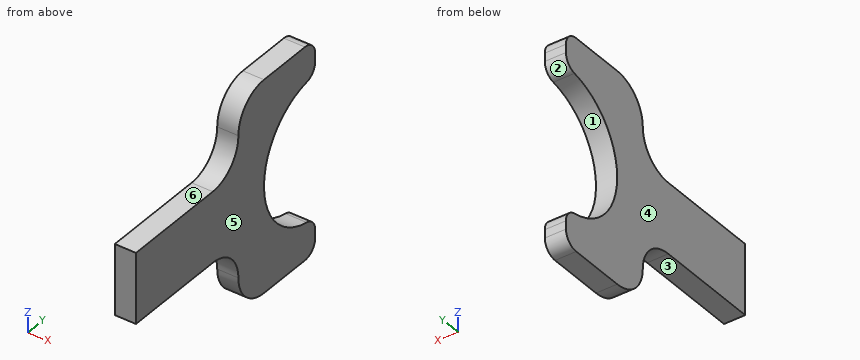
```python
from build123d import *

# Parameters (mm, degrees)
SKETCH1_W           = 30
SKETCH1_H           = 35
BOSS_EXTRUDE1_DEPTH = 3
SKETCH2_W           = 10
SKETCH2_H           = 20
CUT_EXTRUDE1_DEPTH  = 3
SKETCH5_R           = 10
CUT_EXTRUDE2_DEPTH  = 3
FILLET1_DEPTH       = 3
FILLET1_2_DEPTH     = 3
FILLET2_R           = 2


with BuildPart() as part:
    # Sketch1 → Boss-Extrude1 (new body)
    with BuildSketch(Plane(origin=(0, 0, 0), x_dir=(0, 0, -1), z_dir=(1, 0, 0))):
        with Locations((15, 17.5)):
            Rectangle(SKETCH1_W, SKETCH1_H)
    extrude(amount=BOSS_EXTRUDE1_DEPTH)

    # Sketch2 → Cut-Extrude1 (cut)
    with BuildSketch(Plane(origin=(3, 0, 0), x_dir=(0, 0, -1), z_dir=(1, 0, 0))):
        with Locations((5, 10)):
            Rectangle(SKETCH2_W, SKETCH2_H)
        with Locations((25, 10)):
            Rectangle(SKETCH2_W, SKETCH2_H)
    extrude(amount=-CUT_EXTRUDE1_DEPTH, mode=Mode.SUBTRACT)

    # Sketch5 → Cut-Extrude2 (cut)
    with BuildSketch(Plane(origin=(3, 0, 0), x_dir=(0, 0, -1), z_dir=(1, 0, 0))):
        with Locations((15, 35)):
            Circle(SKETCH5_R)
    extrude(amount=-CUT_EXTRUDE2_DEPTH, mode=Mode.SUBTRACT)

    # Fillet1: read off the stored shape, not the designer's step
    # Fillet1 outline → Fillet1 (cut)
    with BuildSketch(Plane.YZ):
        with BuildLine():
            ThreePointArc((25, -30), (21.464466094, -28.535533906), (20, -25))
            Line((20, -25), (20, -30))
            Line((20, -30), (25, -30))
        make_face()
        with BuildLine():
            Line((20, 0), (20, -5))
            ThreePointArc((20, -5), (21.464466094, -1.464466094), (25, 0))
            Line((25, 0), (20, 0))
        make_face()
    extrude(amount=FILLET1_DEPTH, mode=Mode.SUBTRACT)

    # Fillet1 2 outline → Fillet1 2 (add)
    with BuildSketch(Plane.YZ):
        with BuildLine():
            Line((20, -20), (15, -20))
            ThreePointArc((15, -20), (18.535533906, -21.464466094), (20, -25))
            Line((20, -25), (20, -20))
        make_face()
        with BuildLine():
            Line((20, -10), (20, -5))
            ThreePointArc((20, -5), (18.535533906, -8.535533906), (15, -10))
            Line((15, -10), (20, -10))
        make_face()
    extrude(amount=FILLET1_2_DEPTH)

    # Fillet2
    fillet2_edges = [part.edges().sort_by_distance(p)[0] for p in [
        (1.5, 35, -25),
        (1.5, 35, -5),
        (1.5, 35, 0),
        (1.5, 35, -30),
    ]]
    fillet(fillet2_edges, radius=FILLET2_R)


solid = part.part
```
Geometry check sheet. Reference: the model listing, model coordinates, mm. Face numbers are marked on the shaded views. A direction names the side the tool comes from. Round coordinates to 2 decimals unless told otherwise and drop trailing zeros. Loops run counter-clockwise (first coordinate to the right, second up) from the corner with the lowest first, then second, coordinate; pieces in that order, holes last. Notation, with made-up numbers: (37, 19) - (72, 19) arc R32 cw to (72, 57) - close; hole circle Ø4 at (32.25, 45). An arc over 180 degrees is marked (long way). Write each question's results on one line, items separated by ' | '. Start each with the question number.
Q1. Cross-section at A-A on y = 27. Enter the section's corners in (x, z).
Q2. Access from +Z, -Z, +X, -X, +Y, -Y to the whole of each face (thin tool, end or side, straight path). Record for the marked faces 5 and 6.
Q3. Cross-section at B-B on x = 0.4. Enter the section's corners in (y, z), and give its area (3 significant figures).
Q4. Cross-section at D-D on y = 32. Enter the section's corners in (x, z), and give its area (3 significant figures).
Q5. Thickness scan on line 1 (Z direction, x = 0.3, y = 12); line 2 (Z direction, x = 1.95, y = 29); line 3 (Z direction, x = 2.2, y = 33). Record the ranges inside material, lowest first. Write a range as [from, to].
Q6. Cross-section at C-C on y = 9. Enter the section's corners in (x, z), and give its area (3 significant figures).
Q7. Gauge pin test, flat ends, axial feed: P1, Ø1.5, axis at x = 0.5, y = 24, coming from the +Z side; P2, Ø1, axis at x = 2.5, z = -21.5, coming from the +Y side; P3, Ø0.9, axis at x = 1, y = 7.5, coming from the +Z side. Record the tip position at first contact, or that the pin passes through.
Q8. Release check for a two-part mould opening along Z. For the marked faces 1, 2, 3 and 4 record: +Z half, -Z half, draft (parallel to the pull), parting line (faces both ways), or undercut.
Answers below:
1) outline: (0, -30) - (3, -30) - (3, -21) - (0, -21) - close; (0, -9) - (3, -9) - (3, 0) - (0, 0) - close
2) face 5: +Z, -Z, +X, +Y, -Y | face 6: +Z, +X, -X, -Y
3) outline: (0, -20) - (15, -20) arc R5 cw to (20, -25) arc R5 ccw to (25, -30) - (33, -30) arc R2 ccw to (35, -28) - (35, -26.83) arc R2 ccw to (33.33, -24.86) arc R10 cw to (33.33, -5.14) arc R2 ccw to (35, -3.17) - (35, -2) arc R2 ccw to (33, 0) - (25, 0) arc R5 ccw to (20, -5) arc R5 cw to (15, -10) - (0, -10) - close | area: 490 mm²
4) outline: (0, -30) - (3, -30) - (3, -24.54) - (0, -24.54) - close; (0, -5.46) - (3, -5.46) - (3, 0) - (0, 0) - close | area: 32.8 mm²
5) line 1: z = [-20, -10] | line 2: z = [-30, -23], [-7, 0] | line 3: z = [-30, -24.8], [-5.2, 0]
6) outline: (0, -20) - (3, -20) - (3, -10) - (0, -10) - close | area: 30.0 mm²
7) P1: stops at z = -0.01 | P2: stops at y = 27.86 | P3: stops at z = -10
8) face 1: undercut | face 2: undercut | face 3: -Z half | face 4: draft
